```python
from build123d import *

# Parameters (mm, degrees)
F1_DEPTH  = 29.811595
F2_R      = 29.029184
F3_DEPTH  = 71.004875
F3_FACE_R = 29.029184
F4_DEPTH  = 292.082846


with BuildPart() as f1:
    # F0 (on Right) → F1 (new body)
    with BuildSketch(Plane.YZ):
        Polygon((-73.794099, 17.247879), (-51.834151, -55.283625), (21.959948, -72.531504), (73.794099, -17.247879), (51.834151, 55.283625), (-21.959948, 72.531504), align=None)
    extrude(amount=F1_DEPTH)

    # F2 (on Right) → F3 (join)
    with BuildSketch(Plane.YZ):
        with Locations((18.193632, -24.816409)):
            Circle(F2_R)
    extrude(amount=-F3_DEPTH)

    # F3_face (on face) → F4 (join)
    with BuildSketch(Plane(origin=(-71.004875, 18.193632, -24.816409), x_dir=(0, 1, 0), z_dir=(-1, 0, 0))):
        Circle(F3_FACE_R)
    extrude(amount=F4_DEPTH)


solid = f1.part
```
Source: CAD feature listing. Evaluate the final solid. Frame: model axes, mm. A direction names the side the tool comes from. Give positions to 0.01 mm unless a question says otherwise; leave off trailing zeros. Loops run counter-clockwise (first coordinate to the right, second up) from the corner with the lowest first, then second, coordinate; pieces in that order, holes last. Notation, with made-up numbers: (85, 89.5) -> (108, 89.5) arc R14 cw to (108, 93.5) -> close; hole circle Ø10 at (13, 67). An arc over 180 degrees is marked (long way). Use a Markdown table: item, result. Add a question column.
(1) First-contact query: pin 1 Ø4 at (x, z) = (-50.5, 3) entering from -Y; pin 2 Ø5 at (x, y) = (-59, -2.5) entering from +Z; pin 3 Ø8 at (y, z) = (26, 7.5) entering from -X. Flat tips, straight axial feed; report the tip coordinate or a pass-through.
(2) Section query C-C (x = -254.5). Output: boundary loops of the cut face in (y, z), then the cut area to 3 significant figures.
(3) Ray query, line 1 (X direction, y = 56, z = 28.5); line 2 (Y direction, x = -115, z = -26); line 3 (Z direction, x = -20, y = 7.5). Return the intervals inside material, ascending.
(4) Access query for faces 1 (the face through (14.697, -62.968, -18.51)), 2 (the face through (-179, 45.88, -33.54)). Directions: +Z, -Z, +X, -X, +Y, -Y. A direction counts if a zero-diameter tool reaches every point of the face in a straight line with its end or side. Return the directions, or none.
(5) Section query B-B (z = -10.5). Output: boundary loops of the cut face in (x, y).
(6) Section query D-D (z = -61.5). Output: boundary loops of the cut face in (x, y).
(7) Section query A-A (y = 9.5). Output: boundary loops of the cut face in (x, z).
Checked values:
| question | item | result |
|---|---|---|
| 1 | pin 1 | y = 4.92 |
| 1 | pin 2 | z = -2.2 |
| 1 | pin 3 | x = 0 |
| 2 | outline | circle Ø58.06 at (18.19, -24.82) |
| 2 | area | 2,650 mm^2 |
| 3 | line 1 | 0 to 29.81 |
| 3 | line 2 | -10.81 to 47.2 |
| 3 | line 3 | -51.8 to 2.17 |
| 4 | face 1 | -Z, +X, -X, -Y |
| 4 | face 2 | -X |
| 5 | outline | (-363.09, -7.06) -> (0, -7.06) -> (0, -65.39) -> (29.81, -65.39) -> (29.81, 71.75) -> (0, 71.75) -> (0, 43.45) -> (-363.09, 43.45) -> close |
| 6 | outline | (0, -25.24) -> (29.81, -25.24) -> (29.81, 32.3) -> (0, 32.3) -> close |
| 7 | outline | (-363.09, -52.51) -> (0, -52.51) -> (0, -69.62) -> (29.81, -69.62) -> (29.81, 65.18) -> (0, 65.18) -> (0, 2.88) -> (-363.09, 2.88) -> close |
